from build123d import *

# Parameters (mm, degrees)
SKETCH_1_R          = 1.65
SKETCH_1_R_2        = 1.5
EXTRUDE_1_DEPTH     = 3
FILLET_1_R          = 2
EXTRUDE_2_DEPTH     = 3
FILLET_2_R          = 10
SKETCH_3_W          = 43
SKETCH_3_H          = 4
EXTRUDE_3_DEPTH     = 3
FILLET_3_R          = 5
SKETCH_4_W          = 43
SKETCH_4_H          = 19.849699933
CUT_EXTRUDE_1_DEPTH = 10
FILLET_4_R          = 3
FILLET_5_R          = 3
FILLET_6_R          = 3
FILLET_7_R          = 3


with BuildPart() as part:
    # 草图1 → 凸台-拉伸1 (new body)
    with BuildSketch(Plane(origin=(0, 0, 0), x_dir=(1, 0, 0), z_dir=(0, 1, 0))):
        with BuildLine():
            Line((-37, 3), (-35, 3))
            ThreePointArc((-35, 3), (-27.928932188, 5.928932188), (-25, 13))
            Line((-25, 13), (-25, 42))
            ThreePointArc((-25, 42), (-24.121320344, 44.121320344), (-22, 45))
            Line((-22, 45), (22, 45))
            ThreePointArc((22, 45), (24.121320344, 44.121320344), (25, 42))
            Line((25, 42), (25, 13))
            ThreePointArc((25, 13), (27.928932188, 5.928932188), (35, 3))
            Line((35, 3), (37, 3))
            ThreePointArc((37, 3), (38.414213562, 2.414213562), (39, 1))
            Line((39, 1), (39, -1))
            ThreePointArc((39, -1), (38.414213562, -2.414213562), (37, -3))
            Line((37, -3), (35, -3))
            ThreePointArc((35, -3), (27.928932188, -5.928932188), (25, -13))
            Line((25, -13), (25, -27))
            ThreePointArc((25, -27), (24.414213562, -28.414213562), (23, -29))
            Line((23, -29), (-0.329591816, -29))
            Line((-0.329591816, -29), (-23, -29))
            ThreePointArc((-23, -29), (-24.414213562, -28.414213562), (-25, -27))
            Line((-25, -27), (-25, -13))
            ThreePointArc((-25, -13), (-27.928932188, -5.928932188), (-35, -3))
            Line((-35, -3), (-37, -3))
            ThreePointArc((-37, -3), (-38.414213562, -2.414213562), (-39, -1))
            Line((-39, -1), (-39, 1))
            ThreePointArc((-39, 1), (-38.414213562, 2.414213562), (-37, 3))
        make_face()
        with Locations((35, 0)):
            Circle(SKETCH_1_R, mode=Mode.SUBTRACT)
        with Locations((-35, 0)):
            Circle(SKETCH_1_R, mode=Mode.SUBTRACT)
        with Locations((21, 38)):
            Circle(SKETCH_1_R_2, mode=Mode.SUBTRACT)
        with Locations((21, -25)):
            Circle(SKETCH_1_R_2, mode=Mode.SUBTRACT)
        with Locations((-21, 38)):
            Circle(SKETCH_1_R_2, mode=Mode.SUBTRACT)
        with Locations((-21, -25)):
            Circle(SKETCH_1_R_2, mode=Mode.SUBTRACT)
        Polygon((-16.5, 42), (16.5, 42), (16.5, 35.7), (22, 35.7), (22, -22.7), (15.5, -22.7), (15.5, -27), (-15.5, -27), (-15.5, -22.7), (-21, -22.7), (-21, 35.7), (-16.5, 35.7), align=None, mode=Mode.SUBTRACT)
    extrude(amount=EXTRUDE_1_DEPTH)

    # 圆角1
    fillet_1_edges = [part.edges().sort_by_distance(p)[0] for p in [
        (-16.5, 1.5, -42),
        (-21, 1.5, -35.7),
        (-21, 1.5, 22.7),
        (-15.5, 1.5, 27),
        (15.5, 1.5, 27),
        (22, 1.5, 22.7),
        (22, 1.5, -35.7),
        (16.5, 1.5, -42),
    ]]
    fillet(fillet_1_edges, radius=FILLET_1_R)

    # 草图2 → 凸台-拉伸2 (add)
    with BuildSketch(Plane(origin=(0, 3, 0), x_dir=(1, 0, 0), z_dir=(0, 1, 0))):
        with BuildLine():
            Line((36, -3), (25, -20))
            Line((25, -20), (25, -13))
            ThreePointArc((25, -13), (27.928932188, -5.928932188), (35, -3))
            Line((35, -3), (36, -3))
        make_face()
        with BuildLine():
            Line((-25, -13), (-25, -20))
            Line((-25, -20), (-36, -3))
            Line((-36, -3), (-35, -3))
            ThreePointArc((-35, -3), (-27.928932188, -5.928932188), (-25, -13))
        make_face()
    extrude(amount=-EXTRUDE_2_DEPTH)

    # 圆角2
    fillet_2_edges = [part.edges().sort_by_distance(p)[0] for p in [
        (36, 1.5, 3),
        (25, 1.5, 20),
        (-36, 1.5, 3),
        (-25, 1.5, 20),
    ]]
    fillet(fillet_2_edges, radius=FILLET_2_R)

    # 草图3 → 凸台-拉伸3 (add)
    with BuildSketch(Plane(origin=(0, 3, 0), x_dir=(1, 0, 0), z_dir=(0, 1, 0))):
        with Locations((0.5, 8.5)):
            Rectangle(SKETCH_3_W, SKETCH_3_H)
    extrude(amount=-EXTRUDE_3_DEPTH)

    # 圆角3
    fillet_3_edges = [part.edges().sort_by_distance(p)[0] for p in [
        (-21, 1.5, -6.5),
        (22, 1.5, -6.5),
        (22, 1.5, -10.5),
        (-21, 1.5, -10.5),
    ]]
    fillet(fillet_3_edges, radius=FILLET_3_R)

    # 草图4 → 切除-拉伸1 (cut)
    with BuildSketch(Plane(origin=(0, 3, 0), x_dir=(1, 0, 0), z_dir=(0, 1, 0))):
        with Locations((0.5, 9.924849967)):
            Rectangle(SKETCH_4_W, SKETCH_4_H)
    extrude(amount=-CUT_EXTRUDE_1_DEPTH, mode=Mode.SUBTRACT)

    # 圆角4
    fillet_4_edges = [part.edges().sort_by_distance(p)[0] for p in [
        (16.5, 1.5, -35.7),
    ]]
    fillet(fillet_4_edges, radius=FILLET_4_R)

    # 圆角5
    fillet_5_edges = [part.edges().sort_by_distance(p)[0] for p in [
        (-16.5, 1.5, -35.7),
    ]]
    fillet(fillet_5_edges, radius=FILLET_5_R)

    # 圆角6
    fillet_6_edges = [part.edges().sort_by_distance(p)[0] for p in [
        (-15.5, 1.5, 22.7),
    ]]
    fillet(fillet_6_edges, radius=FILLET_6_R)

    # 圆角7
    fillet_7_edges = [part.edges().sort_by_distance(p)[0] for p in [
        (15.5, 1.5, 22.7),
    ]]
    fillet(fillet_7_edges, radius=FILLET_7_R)


solid = part.part
Part model, mm, in its own coordinate system. A direction names the side the tool comes from. Round coordinates to 2 decimals unless told otherwise and drop trailing zeros. Write each loop counter-clockwise with the first axis right and the second up, starting at its lowest first coordinate (ties: lowest second). Pieces come first, ordered by that corner, then holes. Notation, with made-up numbers: (-4, -34.5) - (32, -34.5) arc R24 cw to (32, 4.5) - close; hole circle Ø11 at (18, -36). An arc over 180 degrees is marked (long way). Use CSV: the item, a comma, the result in double quotes.
Item 1: Tool access for faces 4 (the flat face through (-25, 1, -27)), 5 (the flat face through (25, 1, -28)), 6 (the cylindrical face through (21.43, 1.52, 22.1)), 7 (the flat face through (0, 1, -45)): list every direction of +Z, -Z, +X, -X, +Y, -Y with a clear straight run to the whole face (end or side of a thin tool).
Results list:
face 4,"-Z, -X, +Y, -Y"
face 5,"-Z, +X, +Y, -Y"
face 6,"+Y, -Y"
face 7,"-Z, +X, -X, +Y, -Y"
Item 2: Pull direction X, two halves, no side cores. Call faces 1 (the flat face through (0, 1, 29)), 2 (the cylindrical face through (33.35, 1.48, -0.07)), 3 (the cylindrical face through (38.7, 1.48, 2.05)): pulls with the +X half, pulls with the -X half, needs draft (parallel to the pull), parting line crosses it, or undercut.
Results list:
face 1,"needs draft"
face 2,"undercut"
face 3,"pulls with the +X half"
Item 3: Flat gauge pins, fed straight in: P1, Ø1.5, axis at y = 1.5, z = -23, coming from the +X side; P2, Ø0.6, axis at x = 36, y = 1.5, coming from the -Z side; P3, Ø4, axis at x = 17, z = 19.5, coming from the -Y side; P4, Ø0.9, axis at y = 2, z = -11, coming from the +X side. Where does each tip first touch, or does it go through?
Results list:
P1,"stops at x = 25"
P2,"stops at z = -3"
P3,"passes through"
P4,"stops at x = 25.3"
Item 4: Slice it at C-C, the plane x = 21. Write the cut outline in (y, z), then the cut area to 3 significant figures.
Results list:
outline,"(0, -45) - (3, -45) - (3, -39.5) - (0, -39.5) - close; (0, -36.5) - (3, -36.5) - (3, -35.43) - (0, -35.43) - close; (0, 22.43) - (3, 22.43) - (3, 23.5) - (0, 23.5) - close; (0, 26.5) - (3, 26.5) - (3, 29) - (0, 29) - close"
area,"30.4 mm²"
Item 5: Wall check: L1, parallel to X at y = 0.25, z = -26; L2, parallel to X at y = 0.9, z = 25; L3, parallel to X at y = 0.25, z = 24. Give the ranges that are in metal, low to high.
Results list:
L1,"x = -25 to -21, 22 to 25"
L2,"x = -25 to -22.5, -19.5 to -15.53, 15.53 to 19.5, 22.5 to 25"
L3,"x = -25 to -22.12, -19.88 to -15.98, 15.98 to 19.88, 22.12 to 25"
Item 6: Slice it at A-A, the plane z = 0. Write the cut outline in (x, y).
Results list:
outline,"(-39, 0) - (-36.65, 0) - (-36.65, 3) - (-39, 3) - close; (-33.35, 0) - (-21, 0) - (-21, 3) - (-33.35, 3) - close; (22, 0) - (33.35, 0) - (33.35, 3) - (22, 3) - close; (36.65, 0) - (39, 0) - (39, 3) - (36.65, 3) - close"
Item 7: Slice it at B-B, the plane z = 13. Write the cut outline in (x, y).
Results list:
outline,"(-29.53, 0) - (-21, 0) - (-21, 3) - (-29.53, 3) - close; (22, 0) - (29.53, 0) - (29.53, 3) - (22, 3) - close"
Item 8: Slice it at D-D, the plane y = 0.85. Count the separate pieces of the cut face and the enclosed holes in it, then the cut area to 3 significant figures.
Results list:
separate pieces,"1"
enclosed holes,"7"
area,"1,200 mm²"
